```python
from build123d import *

# Parameters (mm, degrees)
F1_DEPTH = 50
F2_DEPTH = 5
F3_W     = 20
F3_H     = 2
F4_DEPTH = 5


with BuildPart() as f1:
    # F0 (on Front) → F1 (new body)
    with BuildSketch(Plane.XZ):
        Polygon((0, 30), (0, 0), (40, 0), (40, 30), (30, 30), (30, 13.209878), (10, 13.209878), (10, 30), align=None)
    extrude(amount=F1_DEPTH)

    # F1_face (on face) → F2 (join)
    with BuildSketch(Plane(origin=(20, -50, 12.43351), x_dir=(1, 0, 0), z_dir=(0, -1, 0))):
        Polygon((10, 0.776368), (-10, 0.776368), (-10, 17.56649), (-20, 17.56649), (-20, -12.43351), (20, -12.43351), (20, 17.56649), (10, 17.56649), align=None)
    extrude(amount=F2_DEPTH)

    # F3 (on Front) → F4 (join)
    with BuildSketch(Plane.XZ):
        with Locations((19.894101, 17.3732)):
            Rectangle(F3_W, F3_H)
        with Locations((19.894101, 22.438831)):
            Rectangle(F3_W, F3_H)
        with Locations((19.894101, 26.903864)):
            Rectangle(F3_W, F3_H)
    extrude(amount=F4_DEPTH)


solid = f1.part
```
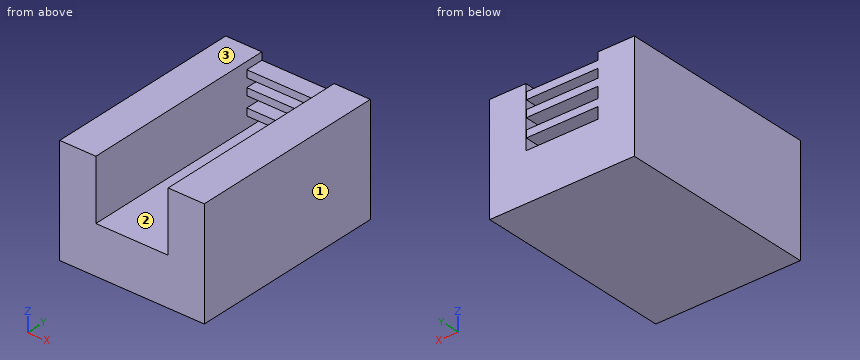
Verification items for the finished model (mm, model axes). Face numbers are marked on the shaded views. Round coordinates to 2 decimals unless told otherwise and drop trailing zeros. Order: outer loops, then holes, each group sorted by start corner. A loop starts at its lowest first (then second) coordinate and runs counter-clockwise, first axis right, second up. Notation, with made-up numbers: (-27, 79.25) -> (-12, 79.25) arc R25 ccw to (-12, 115.25) -> close; hole circle Ø11 at (-24, 12). An arc over 180 degrees is marked (long way). Put each result on its own line as item: value. Start each with the question number.
(1) Depth check by flat-ended pin: pin 1 Ø1.5 at (x, y) = (25, -2) entering from +Z; pin 2 Ø1 at (x, z) = (22.5, 22.5) entering from -Y; pin 3 Ø10 at (x, y) = (23.5, -21.5) entering from +Z. Enter the tip coordinate at first touch or a pass-through.
(2) Draft check along X on the marked faces 1, 2 and 3. Enter one of: +X half, -X half, draft (parallel to the pull), parting line (faces both ways), or undercut.
(3) Section check A-A (x = 20). Enter the section's corners in (y, z).
(4) Section check B-B (z = 24.5). Enter the section's corners in (x, y).
(5) Material ranges on line 1 along Z through (x, y) = (11.5, -2.5); line 2 along X through (y, z) = (-13.5, 15); line 3 along Z through (x, y) = (21.5, -28), recorded low to high.
(6) Section check C-C (y = -6.5). Enter the section's corners in (x, z), then the cut area to 3 significant figures.
Completed:
1. pin 1: stops at z = 27.9
1. pin 2: stops at y = -5
1. pin 3: stops at z = 13.21
2. face 1: +X half
2. face 2: undercut
2. face 3: draft
3. outline: (-55, 0) -> (0, 0) -> (0, 13.21) -> (-55, 13.21) -> close; (-5, 16.37) -> (0, 16.37) -> (0, 18.37) -> (-5, 18.37) -> close; (-5, 21.44) -> (0, 21.44) -> (0, 23.44) -> (-5, 23.44) -> close; (-5, 25.9) -> (0, 25.9) -> (0, 27.9) -> (-5, 27.9) -> close
4. outline: (0, -55) -> (10, -55) -> (10, 0) -> (0, 0) -> close; (30, -55) -> (40, -55) -> (40, 0) -> (30, 0) -> close
5. line 1: z = 0 to 13.21, 16.37 to 18.37, 21.44 to 23.44, 25.9 to 27.9
5. line 2: x = 0 to 10, 30 to 40
5. line 3: z = 0 to 13.21
6. outline: (0, 0) -> (40, 0) -> (40, 30) -> (30, 30) -> (30, 13.21) -> (10, 13.21) -> (10, 30) -> (0, 30) -> close
6. area: 864 mm2
